```python
from build123d import *

# Parameters (mm, degrees)
SKETCH1_R           = 3.1
BOSS_EXTRUDE1_DEPTH = 4.5


with BuildPart() as part:
    # Sketch1 → Boss-Extrude1 (new body)
    with BuildSketch(Plane(origin=(0, 0, 0), x_dir=(1, 0, 0), z_dir=(0, 1, 0))):
        with BuildLine():
            Line((-30, -12.5), (39, -12.5))
            ThreePointArc((39, -12.5), (39.707106781, -12.207106781), (40, -11.5))
            Line((40, -11.5), (40, 12.5))
            Line((40, 12.5), (35, 12.5))
            Line((35, 12.5), (35, 16))
            ThreePointArc((35, 16), (34.707106781, 16.707106781), (34, 17))
            Line((34, 17), (21, 17))
            ThreePointArc((21, 17), (20.292893219, 16.707106781), (20, 16))
            Line((20, 16), (20, 12.5))
            Line((20, 12.5), (15, 12.5))
            Line((15, 12.5), (15, 16))
            ThreePointArc((15, 16), (14.707106781, 16.707106781), (14, 17))
            Line((14, 17), (1, 17))
            ThreePointArc((1, 17), (0.292893219, 16.707106781), (0, 16))
            Line((0, 16), (0, 12.5))
            Line((0, 12.5), (-30, 12.5))
            ThreePointArc((-30, 12.5), (-37.071067812, 9.571067812), (-40, 2.5))
            Line((-40, 2.5), (-40, -2.5))
            ThreePointArc((-40, -2.5), (-37.071067812, -9.571067812), (-30, -12.5))
        make_face()
        with Locations(Location((-30, 0, 0), (0, 0, 270))):
            Circle(SKETCH1_R, mode=Mode.SUBTRACT)
    extrude(amount=BOSS_EXTRUDE1_DEPTH)


solid = part.part
```
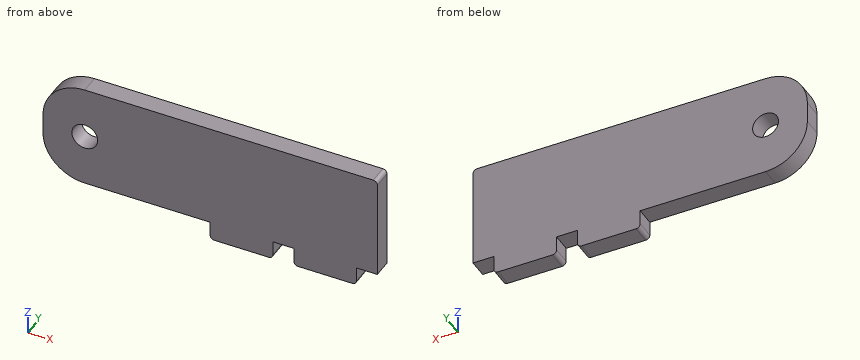
Model file for the job. Use its own axes, mm. Round coordinates to 2 decimals unless told otherwise and drop trailing zeros. Order: outer loops, then holes, each group sorted by start corner. A loop starts at its lowest first (then second) coordinate and runs counter-clockwise, first axis right, second up. Notation, with made-up numbers: (77.5, -38.75) -> (125.5, -38.75) arc R10 cw to (125.5, -34.75) -> close; hole circle Ø6 at (67.5, 13.25). An arc over 180 degrees is marked (long way). Use one line per item in the form item = value.
Item 1: Cut at A-A, the plane z = -13.5. Write the cut outline in (x, y), and give its area (3 significant figures).
Returned:
outline = (0, 0) -> (15, 0) -> (15, 4.5) -> (0, 4.5) -> close; (20, 0) -> (35, 0) -> (35, 4.5) -> (20, 4.5) -> close
area = 135 mm^2
Item 2: Cut at D-D, the plane z = 0. Write the cut outline in (x, y).
Returned:
outline = (-40, 0) -> (-33.1, 0) -> (-33.1, 4.5) -> (-40, 4.5) -> close; (-26.9, 0) -> (40, 0) -> (40, 4.5) -> (-26.9, 4.5) -> close
Item 3: Flat gauge pins, fed straight in: pin 1 Ø1.3 at (x, y) = (18, 2) entering from -Z; pin 2 Ø5 at (x, z) = (-30, 0) entering from -Y; pin 3 Ø8 at (x, z) = (-31.5, 0.5) entering from +Y; pin 4 Ø1 at (y, z) = (1.5, -15) entering from +X. Where does each tip first touch, or does it go through?
Returned:
pin_1 = -12.5
pin_2 = through
pin_3 = 4.5
pin_4 = 35
Item 4: Cut at B-B, the plane y = 1.55. Write the cut outline in (x, z).
Returned:
outline = (-40, -2.5) arc R10 ccw to (-30, -12.5) -> (0, -12.5) -> (0, -16) arc R1 ccw to (1, -17) -> (14, -17) arc R1 ccw to (15, -16) -> (15, -12.5) -> (20, -12.5) -> (20, -16) arc R1 ccw to (21, -17) -> (34, -17) arc R1 ccw to (35, -16) -> (35, -12.5) -> (40, -12.5) -> (40, 11.5) arc R1 ccw to (39, 12.5) -> (-30, 12.5) arc R10 ccw to (-40, 2.5) -> close; hole circle Ø6.2 at (-30, 0)
Item 5: Drill centre lines: line 1 (X direction, y = 1.3, z = 0); line 2 (X direction, y = 2.05, z = -15.5); line 3 (Z direction, x = -11.5, y = 0.25). Where is each one in solid material? Low to high.
Returned:
line_1 = -40 to -33.1, -26.9 to 40
line_2 = 0 to 15, 20 to 35
line_3 = -12.5 to 12.5
Item 6: Cut at C-C, the plane x = -1.5. Write the cut outline in (y, z).
Returned:
outline = (0, -12.5) -> (4.5, -12.5) -> (4.5, 12.5) -> (0, 12.5) -> close
